For this review, take the finished solid that the model builds, in its own axes (mm). A direction names the side the tool comes from. Coordinates: 2 decimals unless noted, no trailing zeros. Order: outer loops, then holes, each group sorted by start corner. A loop starts at its lowest first (then second) coordinate and runs counter-clockwise, first axis right, second up.
from build123d import *

# Parameters (mm, degrees)
SKETCH_R      = 70
PAD_DEPTH     = 70
SKETCH001_R   = 50
SKETCH001_R_2 = 40
PAD001_DEPTH  = 50


with BuildPart() as part:
    # Sketch → Pad (new body)
    with BuildSketch(Plane.XY):
        with Locations((90, 70)):
            Circle(SKETCH_R)
    extrude(amount=PAD_DEPTH)

    # Sketch001 (on Face3 of Pad) → Pad001 (join)
    with BuildSketch(Plane.XY.offset(70)):
        with Locations((90, 70)):
            Circle(SKETCH001_R)
        with Locations((90, 70)):
            Circle(SKETCH001_R_2, mode=Mode.SUBTRACT)
    extrude(amount=PAD001_DEPTH)


solid = part.part
1. Take a section at C-C, the plane z = 73. Give the boundary of the cut face in (x, y), plus the area to 3 significant figures.
Answer below:
outline: circle Ø100 at (90, 70); hole circle Ø80 at (90, 70)
area: 2,830 mm2
2. Clearance check with flat-ended pins moving along their axes: pin 1 Ø1 at (x, y) = (88.5, 65) entering from +Z; pin 2 Ø12 at (x, z) = (93, 33) entering from +Y; pin 3 Ø5 at (y, z) = (44, 85) entering from +X; pin 4 Ø8 at (x, y) = (139.5, 107) entering from -Z. State where each tip first meets the part, or that it passes through.
Answer below:
pin 1: stops at z = 70
pin 2: stops at y = 140
pin 3: stops at x = 134.13
pin 4: stops at z = 0
3. Take a section at D-D, the plane z = 25.5. Give the boundary of the cut face in (x, y).
Answer below:
outline: circle Ø140 at (90, 70)
4. Take a section at B-B, the plane y = 70. Give the boundary of the cut face in (x, z), plus the area to 3 significant figures.
Answer below:
outline: (20, 0) - (160, 0) - (160, 70) - (140, 70) - (140, 120) - (130, 120) - (130, 70) - (50, 70) - (50, 120) - (40, 120) - (40, 70) - (20, 70) - close
area: 10,800 mm2
5. Take a section at A-A, the plane x = 90. Give the boundary of the cut face in (y, z).
Answer below:
outline: (0, 0) - (140, 0) - (140, 70) - (120, 70) - (120, 120) - (110, 120) - (110, 70) - (30, 70) - (30, 120) - (20, 120) - (20, 70) - (0, 70) - close
6. To check wall thickness, follow L1, parallel to X at y = 69.5, z = 72.5; L2, parallel to Y at x = 90, z = 109; L3, parallel to Z at x = 112, y = 115. State the ranges of each line that lie inside material, in increasing order.
Answer below:
L1: x = 40 to 50, 130 to 140
L2: y = 20 to 30, 110 to 120
L3: z = 0 to 70
7. Machinability: for faces 4 (the face through (89, 71, 70)), 5 (the face through (89, 71, 0)), which of the approach directions +Z, -Z, +X, -X, +Y, -Y give a long, thin tool a straight path to every point of the face, cutting with its end or side? Answer none if there is none.
Answer below:
face 4: +Z
face 5: -Z, +X, -X, +Y, -Y
8. The part is to be moulded in two halves that separate along X. For faces 1 (the face through (68, 104, 120)), 2 (the face through (80.887, 139.404, 34.51)), 3 (the face through (128.153, 82.015, 94.65)), say which applies: +X half, -X half, draft (parallel to the pull), parting line (faces both ways), or undercut.
Answer below:
face 1: draft
face 2: parting line
face 3: undercut
